The model under review builds one solid part; all positions refer to its coordinate system, in mm. A direction names the side the tool comes from. Round coordinates to 2 decimals unless told otherwise and drop trailing zeros. Order: outer loops, then holes, each group sorted by start corner. A loop starts at its lowest first (then second) coordinate and runs counter-clockwise, first axis right, second up. Notation, with made-up numbers: (15.25, 65) -> (48.25, 65) arc R17 ccw to (48.25, 89) -> close; hole circle Ø10 at (-25.75, 39). An arc over 180 degrees is marked (long way). Use a Markdown table: item, result. Add a question column.
```python
from build123d import *

# Parameters (mm, degrees)
SKETCH_1_W           = 19
SKETCH_1_H           = 19
SKETCH_1_W_2         = 13
SKETCH_1_H_2         = 13
EXTRUDE_2_DEPTH      = 20.4
SKETCH_1_3_W         = 19
SKETCH_1_3_H         = 19
SKETCH_1_3_W_2       = 16.2
SKETCH_1_3_H_2       = 16.2
CUT_EXTRUDE_1_DEPTH  = 17.4
EXTRUDE_4_DEPTH      = 26.65
CUT_EXTRUDE_4_DEPTH  = 11.65
CUT_EXTRUDE_9_DEPTH  = 2
CUT_EXTRUDE_10_DEPTH = 2
CUT_EXTRUDE_11_DEPTH = 2
CUT_EXTRUDE_12_DEPTH = 2
SKETCH_12_W          = 39
SKETCH_12_H          = 3.5
CUT_EXTRUDE_13_DEPTH = 4


with BuildPart() as part:
    # Sketch 1 → Extrude 2 (new body, symmetric)
    with BuildSketch(Plane.XY):
        Rectangle(SKETCH_1_W, SKETCH_1_H)
        Rectangle(SKETCH_1_W_2, SKETCH_1_H_2, mode=Mode.SUBTRACT)
    extrude(amount=EXTRUDE_2_DEPTH, both=True)

    # Sketch 1_3 → Cut-Extrude 1 (cut, symmetric)
    with BuildSketch(Plane.XY):
        Rectangle(SKETCH_1_3_W, SKETCH_1_3_H)
        Rectangle(SKETCH_1_3_W_2, SKETCH_1_3_H_2, mode=Mode.SUBTRACT)
    extrude(amount=CUT_EXTRUDE_1_DEPTH, both=True, mode=Mode.SUBTRACT)

    # Sketch 2 → Extrude 4 (add, symmetric)
    with BuildSketch(Plane.XY):
        Polygon((-22.5, -16.5), (22.5, -16.5), (22.5, -9.5), (0, -9.5), (-22.5, -9.5), align=None)
    extrude(amount=EXTRUDE_4_DEPTH, both=True)

    # Sketch 2_6 → Cut-Extrude 4 (cut, symmetric)
    with BuildSketch(Plane.XY):
        Polygon((-22.5, -16.5), (22.5, -16.5), (22.5, -9.5), (0, -9.5), (-22.5, -9.5), align=None)
    extrude(amount=CUT_EXTRUDE_4_DEPTH, both=True, mode=Mode.SUBTRACT)

    # Sketch 4 → Cut-Extrude 9 (cut)
    with BuildSketch(Plane(origin=(0, 0, -26.65), x_dir=(-1, 0, 0), z_dir=(0, 0, -1))):
        Polygon((-6, -12.5), (-6, -16.5), (-4, -16.5), (-4, -12.5), (-2.5, -12.5), (-1, -12.5), (-1, -16.5), (1, -16.5), (1, -12.5), (2.5, -12.5), (4, -12.5), (4, -16.5), (6, -16.5), (6, -12.5), (7.5, -12.5), (9, -12.5), (9, -16.5), (11, -16.5), (11, -12.5), (12.5, -12.5), (14, -12.5), (14, -16.5), (16, -16.5), (16, -12.5), (17.5, -12.5), (19, -12.5), (19, -16.5), (22.5, -16.5), (22.5, -9.5), (-22.5, -9.5), (-22.5, -16.5), (-19, -16.5), (-19, -12.5), (-17.5, -12.5), (-16, -12.5), (-16, -16.5), (-14, -16.5), (-14, -12.5), (-12.5, -12.5), (-11, -12.5), (-11, -16.5), (-9, -16.5), (-9, -12.5), (-7.5, -12.5), align=None)
    extrude(amount=-CUT_EXTRUDE_9_DEPTH, mode=Mode.SUBTRACT)

    # Sketch 9 → Cut-Extrude 10 (cut)
    with BuildSketch(Plane.XY.offset(-11.65)):
        Polygon((-4, -12.5), (-1, -12.5), (-1, -16.5), (1, -16.5), (1, -12.5), (4, -12.5), (4, -16.5), (6, -16.5), (6, -12.5), (9, -12.5), (9, -16.5), (11, -16.5), (11, -12.5), (14, -12.5), (14, -16.5), (16, -16.5), (16, -12.5), (19, -12.5), (19, -16.5), (22.5, -16.5), (22.5, -9.5), (-22.5, -9.5), (-22.5, -16.5), (-19, -16.5), (-19, -12.5), (-16, -12.5), (-16, -16.5), (-14, -16.5), (-14, -12.5), (-11, -12.5), (-11, -16.5), (-9, -16.5), (-9, -12.5), (-6, -12.5), (-6, -16.5), (-4, -16.5), align=None)
    extrude(amount=-CUT_EXTRUDE_10_DEPTH, mode=Mode.SUBTRACT)

    # Sketch 10 → Cut-Extrude 11 (cut)
    with BuildSketch(Plane(origin=(0, 0, 11.65), x_dir=(-1, 0, 0), z_dir=(0, 0, -1))):
        Polygon((1, -16.5), (1, -12.5), (4, -12.5), (4, -16.5), (6, -16.5), (6, -12.5), (9, -12.5), (9, -16.5), (11, -16.5), (11, -12.5), (14, -12.5), (14, -16.5), (16, -16.5), (16, -12.5), (19, -12.5), (19, -16.5), (22.5, -16.5), (22.5, -9.5), (-22.5, -9.5), (-22.5, -16.5), (-19, -16.5), (-19, -12.5), (-16, -12.5), (-16, -16.5), (-14, -16.5), (-14, -12.5), (-11, -12.5), (-11, -16.5), (-9, -16.5), (-9, -12.5), (-6, -12.5), (-6, -16.5), (-4, -16.5), (-4, -12.5), (-1, -12.5), (-1, -16.5), align=None)
    extrude(amount=-CUT_EXTRUDE_11_DEPTH, mode=Mode.SUBTRACT)

    # Sketch 11 → Cut-Extrude 12 (cut)
    with BuildSketch(Plane.XY.offset(26.65)):
        Polygon((-1, -12.5), (-1, -16.5), (1, -16.5), (1, -12.5), (4, -12.5), (4, -16.5), (6, -16.5), (6, -12.5), (9, -12.5), (9, -16.5), (11, -16.5), (11, -12.5), (14, -12.5), (14, -16.5), (16, -16.5), (16, -12.5), (19, -12.5), (19, -16.5), (22.5, -16.5), (22.5, -9.5), (-22.5, -9.5), (-22.5, -16.5), (-19, -16.5), (-19, -12.5), (-16, -12.5), (-16, -16.5), (-14, -16.5), (-14, -12.5), (-11, -12.5), (-11, -16.5), (-9, -16.5), (-9, -12.5), (-6, -12.5), (-6, -16.5), (-4, -16.5), (-4, -12.5), align=None)
    extrude(amount=-CUT_EXTRUDE_12_DEPTH, mode=Mode.SUBTRACT)

    # Sketch 12 → Cut-Extrude 13 (cut)
    with BuildSketch(Plane.XZ.offset(16.5)):
        with Locations((0, -21.65)):
            Rectangle(SKETCH_12_W, SKETCH_12_H)
        with Locations((0, 16.65)):
            Rectangle(SKETCH_12_W, SKETCH_12_H)
        with Locations((0, -16.65)):
            Rectangle(SKETCH_12_W, SKETCH_12_H)
        with Locations((0, 21.65)):
            Rectangle(SKETCH_12_W, SKETCH_12_H)
    extrude(amount=-CUT_EXTRUDE_13_DEPTH, mode=Mode.SUBTRACT)


solid = part.part
```
Q1. Mouldability with a two-part tool opening along X and no side actions: class faces 4 (the flat face through (22.5, -13, 19)), 5 (the flat face through (2, -14, 26.65)), 6 (the flat face through (-1, -14, -13)), 7 (the flat face through (-8.1, 0, 0)) as pulls with the +X half, pulls with the -X half, needs draft (parallel to the pull), parting line crosses it, or undercut.
Q2. Add section A-A (x = 15). Write out the cut boundary in (y, z).
Q3. Wall thickness on line 1 (Y direction, x = -5.5, z = -17); line 2 (X direction, y = 1, z = 17); line 3 (Z direction, x = 2.5, y = -12): over which ranges is each line inside the solid? List them lowest first. Write a range as [from, to].
Q4. Insertion check: pin 1 (0.6 mm diameter, centred on y = -14, z = 12.5, fed in from -X); pin 2 (12 mm diameter, centred on x = -7.5, y = 1.5, fed in from +Z); pin 3 (2 mm diameter, centred on y = -14, z = 12.5, fed in from +X). Each pin has a flat end and moves straight along its axis. Give the tip position at first contact, or say it passes through.
Q5. Add section C-C (y = 1.25). Write out the cut boundary in (x, z).
Q6. Machinability: for faces 1 (the flat face through (-11, -14, -13)), 2 (the flat face through (19.5, -15, -17)), 3 (the flat face through (1, -15, 26)), which of the approach directions +Z, -Z, +X, -X, +Y, -Y give a long, thin tool a straight path to every point of the face, cutting with its end or side? Answer none if there is none.
Q7. Add section B-B (z = 1). Write out the cut boundary in (x, y).
Q8. Add section D-D (z = -12.5). State how many separate pieces and enclosed holes the cut face has, then the cut area to 3 significant figures.
Report:
| question | item | result |
|---|---|---|
| 1 | face 4 | pulls with the +X half |
| 1 | face 5 | needs draft |
| 1 | face 6 | undercut |
| 1 | face 7 | pulls with the -X half |
| 2 | outline | (-16.5, -24.65) -> (-9.5, -24.65) -> (-9.5, -13.65) -> (-16.5, -13.65) -> (-16.5, -14.9) -> (-12.5, -14.9) -> (-12.5, -18.4) -> (-16.5, -18.4) -> (-16.5, -19.9) -> (-12.5, -19.9) -> (-12.5, -23.4) -> (-16.5, -23.4) -> close; (-16.5, 13.65) -> (-9.5, 13.65) -> (-9.5, 24.65) -> (-16.5, 24.65) -> (-16.5, 23.4) -> (-12.5, 23.4) -> (-12.5, 19.9) -> (-16.5, 19.9) -> (-16.5, 18.4) -> (-12.5, 18.4) -> (-12.5, 14.9) -> (-16.5, 14.9) -> close |
| 3 | line 1 | y = [-12.5, -9.5], [-8.1, -6.5], [6.5, 8.1] |
| 3 | line 2 | x = [-8.1, -6.5], [6.5, 8.1] |
| 3 | line 3 | z = [-24.65, -13.65], [13.65, 24.65] |
| 4 | pin 1 | stops at x = -19 |
| 4 | pin 2 | stops at z = 20.4 |
| 4 | pin 3 | stops at x = 19 |
| 5 | outline | (-9.5, -20.4) -> (-6.5, -20.4) -> (-6.5, 20.4) -> (-9.5, 20.4) -> (-9.5, 17.4) -> (-8.1, 17.4) -> (-8.1, -17.4) -> (-9.5, -17.4) -> close; (6.5, -20.4) -> (9.5, -20.4) -> (9.5, -17.4) -> (8.1, -17.4) -> (8.1, 17.4) -> (9.5, 17.4) -> (9.5, 20.4) -> (6.5, 20.4) -> close |
| 6 | face 1 | +Y, -Y |
| 6 | face 2 | -Y |
| 6 | face 3 | +Z, +Y, -Y |
| 7 | outline | (-8.1, -8.1) -> (8.1, -8.1) -> (8.1, 8.1) -> (-8.1, 8.1) -> close; hole (-6.5, -6.5) -> (6.5, -6.5) -> (6.5, 6.5) -> (-6.5, 6.5) -> close |
| 8 | separate pieces | 9 |
| 8 | enclosed holes | 1 |
| 8 | area | 189 mm² |
